```python
from build123d import *

# Parameters (mm, degrees)
F1_DEPTH = 50.8
F2_W     = 27.847112
F2_H     = 23.205928
F3_DEPTH = 118.98803
F4_R     = 6.728536
F5_DEPTH = 25.4


with BuildPart() as f1:
    # F0 (on Top) → F1 (new body)
    with BuildSketch(Plane.XY):
        with BuildLine():
            Line((-41.568879, 46.714541), (-26.450199, 25.692446))
            ThreePointArc((-26.450199, 25.692446), (-22.246811, -29.407385), (31.918666, -18.463846))
            Line((31.918666, -18.463846), (60.738988, -18.463846))
            Line((60.738988, -18.463846), (60.738988, 18.463846))
            Line((60.738988, 18.463846), (31.918666, 18.463846))
            ThreePointArc((31.918666, 18.463846), (9.793967, 35.549867), (-17.959369, 32.205215))
            Line((-17.959369, 32.205215), (-17.959369, 40.459029))
            Line((-17.959369, 40.459029), (-7.466254, 48.93424))
            Line((-7.466254, 48.93424), (-27.24174, 66.288233))
            Line((-27.24174, 66.288233), (-41.568879, 46.714541))
        make_face()
    extrude(amount=F1_DEPTH)

    # F2 (on face) → F3 (cut)
    with BuildSketch(Plane.XY.offset(50.8)):
        Rectangle(F2_W, F2_H)
    extrude(amount=-F3_DEPTH, mode=Mode.SUBTRACT)

    # F4 (on face) → F5 (cut)
    with BuildSketch(Plane.XY.offset(50.8)):
        with Locations((39.279759, 4.874428)):
            Circle(F4_R)
    extrude(amount=-F5_DEPTH, mode=Mode.SUBTRACT)


solid = f1.part
```
Could you check a few things on this model? Use its own coordinates, in mm. A direction names the side the tool comes from. Round coordinates to 2 decimals unless told otherwise and drop trailing zeros. Order: outer loops, then holes, each group sorted by start corner. A loop starts at its lowest first (then second) coordinate and runs counter-clockwise, first axis right, second up. Notation, with made-up numbers: M 46,4.25 L 54,4.25 A17 ccw 54,22.25 Z; hole C 53,-4.5 d8. An arc over 180 degrees is marked long. One line per question, with ' | ' between items. Start each with the question number.
(1) Suppose I cut it at D-D on x = -34. List the corners of the cut face in (y, z) for me, then the cut area to 3 significant figures.
(2) Suppose I cut it at A-A on z = 11. List the corners of the cut face in (x, y) for me, then the cut area to 3 significant figures.
(3) Suppose I cut it at C-C on y = 0. List the corners of the cut face in (x, z) for me, then the cut area to 3 significant figures.
(4) Thinking about a two-plate mould opening in Y: for faces 5 (the face through (9, 15, 50.8)), 6 (the face through (46, -18.464, 25)), 7 (the face through (0, -11.603, 26)), which applies, +Y half, -Y half, draft (parallel to the pull), parting line (faces both ways), or undercut?
(5) Please list where these lines run through material, in increasing order: line 1 along Y through (x, z) = (-12, 31); line 2 along X through (y, z) = (8, 38.5); line 3 along Y through (x, z) = (38.5, 5).
(6) For P1, Ø3, axis at x = 48, z = 18, coming from the +Y side; P2, Ø2, axis at y = 22, z = 18, coming from the -X side; P3, Ø8, axis at x = 10, z = 45, coming from the +Y side, each with a flat end and sliding along its axis, tell me the tip position at first contact or that it passes through.
(7) Suppose I cut it at B-B on x = 0. List the corners of the cut face in (y, z) for me.
(8) For faces 1 (the face through (-13.924, 0, 26)), 2 (the face through (-34.115, 36.351, 25.044)), 3 (the face through (47, 18.464, 25)), 4 (the face through (-12.786, 44.637, 25.044)), which set-ups out of +Z, -Z, +X, -X, +Y, -Y let a thin tool reach every point of the face, with its end or its side?
Geometry results:
1) outline: M -14.27,0 L 14.27,0 L 14.27,50.8 L -14.27,50.8 Z; M 36.19,0 L 57.06,0 L 57.06,50.8 L 36.19,50.8 Z | area: 2,510 mm²
2) outline: M -41.57,46.71 L -26.45,25.69 A36.87 ccw long 31.92,-18.46 L 60.74,-18.46 L 60.74,18.46 L 31.92,18.46 A36.87 ccw -17.96,32.21 L -17.96,40.46 L -7.47,48.93 L -27.24,66.29 Z; hole M -13.92,-11.6 L 13.92,-11.6 L 13.92,11.6 L -13.92,11.6 Z | area: 5,250 mm²
3) outline: M -36.87,0 L -13.92,0 L -13.92,50.8 L -36.87,50.8 Z; M 13.92,0 L 60.74,0 L 60.74,50.8 L 43.92,50.8 L 43.92,25.4 L 34.64,25.4 L 34.64,50.8 L 13.92,50.8 Z | area: 3,310 mm²
4) face 5: draft | face 6: -Y half | face 7: undercut
5) line 1: -34.87 to -11.6, 11.6 to 34.87, 45.27 to 52.91 | line 2: -36 to -13.92, 13.92 to 33.32, 45.24 to 60.74 | line 3: -18.46 to 18.46
6) P1: y = 18.46 | P2: x = -30.31 | P3: y = 36.38
7) outline: M -36.87,0 L -11.6,0 L -11.6,50.8 L -36.87,50.8 Z; M 11.6,0 L 36.87,0 L 36.87,50.8 L 11.6,50.8 Z
8) face 1: +Z, -Z | face 2: +Z, -Z, -X | face 3: +Z, -Z, +X, +Y | face 4: +Z, -Z, +X
